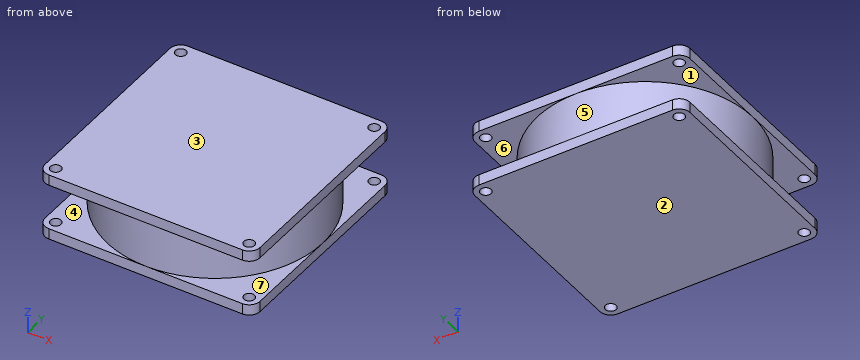
```python
from build123d import *

# Parameters (mm, degrees)
SKETCH1_W             = 80
SKETCH1_H             = 80
BOSS_EXTRUDE1_DEPTH   = 4
FILLET2_R             = 4
SKETCH3_R             = 40
BOSS_EXTRUDE2_DEPTH   = 17
SKETCH4_W             = 80
SKETCH4_H             = 80
BOSS_EXTRUDE3_DEPTH   = 4
FILLET3_R             = 4
F_4_0MM_DOWEL_HOLE1_D = 4


with BuildPart() as part:
    # Sketch1 → Boss-Extrude1 (new body)
    with BuildSketch(Plane.XY):
        with Locations((40, 40)):
            Rectangle(SKETCH1_W, SKETCH1_H)
    extrude(amount=BOSS_EXTRUDE1_DEPTH)

    # Fillet2
    fillet2_edges = [part.edges().sort_by_distance(p)[0] for p in [
        (0, 0, 2),
        (0, 80, 2),
        (80, 80, 2),
        (80, 0, 2),
    ]]
    fillet(fillet2_edges, radius=FILLET2_R)

    # Sketch3 → Boss-Extrude2 (add)
    with BuildSketch(Plane.XY.offset(4)):
        with Locations((40, 40)):
            Circle(SKETCH3_R)
    extrude(amount=BOSS_EXTRUDE2_DEPTH)

    # Sketch4 → Boss-Extrude3 (add)
    with BuildSketch(Plane.XY.offset(21)):
        with Locations((40, 40)):
            Rectangle(SKETCH4_W, SKETCH4_H)
    extrude(amount=BOSS_EXTRUDE3_DEPTH)

    # Fillet3
    fillet3_edges = [part.edges().sort_by_distance(p)[0] for p in [
        (0, 80, 23),
        (0, 0, 23),
        (80, 0, 23),
        (80, 80, 23),
    ]]
    fillet(fillet3_edges, radius=FILLET3_R)

    # Ø4.0mm Dowel Hole1 (through all)
    with Locations(Plane(origin=(0, 0, 0), x_dir=(-1, 0, 0), z_dir=(0, 0, -1))):
        with Locations((-76, 76), (-4, 76), (-4, 4), (-76, 4)):
            Hole(F_4_0MM_DOWEL_HOLE1_D / 2)


solid = part.part
```
The listing builds one solid part. Answer for the finished solid, in the listing's coordinates (mm). Face numbers are marked on the shaded views. A direction names the side the tool comes from. Give positions to 0.01 mm unless a question says otherwise; leave off trailing zeros. Order: outer loops, then holes, each group sorted by start corner. A loop starts at its lowest first (then second) coordinate and runs counter-clockwise, first axis right, second up.
1) Consider line 1 along Y through (x, z) = (4, 23.8); line 2 along Y through (x, z) = (41, 6.75); line 3 along Y through (x, z) = (24, 15.5). Determine where each line is inside the solid, lowest interval first.
Reported:
line 1: y = 0 to 2, 6 to 74, 78 to 80
line 2: y = 0.01 to 79.99
line 3: y = 3.34 to 76.66
2) Find section A-A on x = 64. Write down the section's boundary in (y, z), then the cut area to 3 significant figures.
Reported:
outline: (0, 0) - (80, 0) - (80, 4) - (72, 4) - (72, 21) - (80, 21) - (80, 25) - (0, 25) - (0, 21) - (8, 21) - (8, 4) - (0, 4) - close
area: 1,730 mm2
3) Given P1, Ø3, axis at x = 20, y = 44.5, coming from the -Z side; P2, Ø5, axis at y = 72, z = 7.5, coming from the -X side; P3, Ø6, axis at x = 9.5, z = 13.5, coming from the +Y side; P4, Ø5, axis at x = 54, z = 16, coming from the +Y side, each flat-ended and moving along its own axis, determine where each tip first touches the part or whether it passes through.
Reported:
P1: stops at z = 0
P2: stops at x = 12.99
P3: stops at y = 69.05
P4: stops at y = 78.31
4) For the marked faces 4, 5, 6 and 7, determine the directions among +Z, -Z, +X, -X, +Y, -Y from which every point of the face is accessible in a straight line to the end or side of a thin tool.
Reported:
face 4: -X, -Y
face 5: none
face 6: +X, +Y
face 7: +X, -Y
5) Find section C-C on z = 15.75. Write down the section's boundary in (x, y), then the cut area to 3 significant figures.
Reported:
outline: circle Ø80 at (40, 40)
area: 5,030 mm2
6) Determine the mould class of the marked faces 1, 2 and 3 for opening direction Z: pulls with the +Z half, pulls with the -Z half, needs draft (parallel to the pull), parting line crosses it, or undercut.
Reported:
face 1: undercut
face 2: pulls with the -Z half
face 3: pulls with the +Z half
